from build123d import *

# Parameters (mm, degrees)
SKETCH_1_W          = 20
SKETCH_1_H          = 5
EXTRUDE_1_DEPTH     = 271.75
SKETCH_2_R          = 2.5
CUT_EXTRUDE_1_DEPTH = 125.875
FILLET_1_R          = 10


with BuildPart() as part:
    # 草图1 → 凸台-拉伸1 (new body)
    with BuildSketch(Plane.XY):
        with Locations((7.706454687, 2.403044524)):
            Rectangle(SKETCH_1_W, SKETCH_1_H)
    extrude(amount=EXTRUDE_1_DEPTH)

    # 草图2 → 切除-拉伸1 (cut, symmetric)
    with BuildSketch(Plane(origin=(0, 0, 0), x_dir=(1, 0, 0), z_dir=(0, 1, 0))):
        with Locations((7.706454687, -15)):
            Circle(SKETCH_2_R)
        with Locations((7.706454687, -256.75)):
            Circle(SKETCH_2_R)
    extrude(amount=CUT_EXTRUDE_1_DEPTH, both=True, mode=Mode.SUBTRACT)

    # 圆角1
    fillet_1_edges = [part.edges().sort_by_distance(p)[0] for p in [
        (-2.293545313, 2.403044524, 0),
        (17.706454687, 2.403044524, 0),
        (-2.293545313, 2.403044524, 271.75),
        (17.706454687, 2.403044524, 271.75),
    ]]
    fillet(fillet_1_edges, radius=FILLET_1_R - 0.0001)  # a hair under: the kernel refuses the full size


solid = part.part
The model under review builds one solid part; all positions refer to its coordinate system, in mm. Round coordinates to 2 decimals unless told otherwise and drop trailing zeros. Order: outer loops, then holes, each group sorted by start corner. A loop starts at its lowest first (then second) coordinate and runs counter-clockwise, first axis right, second up. Notation, with made-up numbers: (11, 1.25) -> (62, 1.25) arc R9 ccw to (62, 15.25) -> close; hole circle Ø1 at (88, 72.5). An arc over 180 degrees is marked (long way). Use CSV: the item, a comma, the result in double quotes. Start each with the question number.
(1) Consider section A-A on z = 15. Write out the cut boundary in (x, y).
(2) Wall thickness on probe 1 along Z at (x, y) = (7.5, 0.5); probe 2 along X at (y, z) = (1.6, 15); probe 3 along Z at (x, y) = (10, 4.7): over which ranges is each line inside the solid? List them lowest first. Write a range as from..to.
(3) Consider section C-C on x = 15.5. Write out the cut boundary in (y, z).
(4) Insertion check: pin 1 (4.5 mm diameter, centred on x = 7.71, z = 15, fed in from -Y). The pin has a flat end and moves straight along its axis. Give the tip position at first contact, or say it passes through.
(5) Consider section B-B on y = 2.75. State how many separate pieces and enclosed holes the cut face has, and give its area (3 significant figures).
Responses:
1,outline,"(-2.29, -0.1) -> (5.21, -0.1) -> (5.21, 4.9) -> (-2.29, 4.9) -> close; (10.21, -0.1) -> (17.71, -0.1) -> (17.71, 4.9) -> (10.21, 4.9) -> close"
2,probe 1,"0..12.51, 17.49..254.26, 259.24..271.75"
2,probe 2,"-2.29..5.21, 10.21..17.71"
2,probe 3,"0.27..14.01, 15.99..255.76, 257.74..271.48"
3,outline,"(-0.1, 3.73) -> (4.9, 3.73) -> (4.9, 268.02) -> (-0.1, 268.02) -> close"
4,pin 1,"through"
5,separate pieces,"1"
5,enclosed holes,"2"
5,area,"5,310 mm²"
